For this review, take the finished solid that the model builds, in its own axes (mm). A direction names the side the tool comes from. Round coordinates to 2 decimals unless told otherwise and drop trailing zeros. Loops run counter-clockwise (first coordinate to the right, second up) from the corner with the lowest first, then second, coordinate; pieces in that order, holes last. Notation, with made-up numbers: (56, 58.25) -> (88, 58.25) arc R24 ccw to (88, 76.25) -> close; hole circle Ø5 at (68.25, 82). An arc over 180 degrees is marked (long way). Use one line per item in the form item = value. Start each with the question number.
from build123d import *

# Parameters (mm, degrees)
F1_DEPTH = 127
F2_W     = 101.6
F2_H     = 63.5
F3_DEPTH = 50.8


with BuildPart() as f1:
    # F0 (on Front) → F1 (new body)
    with BuildSketch(Plane.XZ):
        Polygon((-25.4, 95.645057), (-25.4, -5.954943), (127, -5.954943), (127, 95.645057), (101.6, 95.645057), (101.6, 44.845057), (0, 44.845057), (0, 95.645057), align=None)
    extrude(amount=F1_DEPTH)

    # F2 (on face) → F3 (join)
    with BuildSketch(Plane.XY.offset(44.845057)):
        with Locations((50.8, -31.75)):
            Rectangle(F2_W, F2_H)
    extrude(amount=F3_DEPTH)


solid = f1.part
Item 1: For P1, Ø5, axis at x = 72.5, z = 20.5, coming from the +Y side, flat-tipped, find the tip position at first contact; note if it passes through.
Item 2: Draft analysis for pull direction X (two halves, no side actions). For faces 1 (the flat face through (52, -95, 44.845)), 2 (the flat face through (50, -48, 95.645)), 3 (the flat face through (-25.4, -63, 46)), 4 (the flat face through (50, -63.5, 70)), state which applies: +X half, -X half, draft (parallel to the pull), parting line (faces both ways), or undercut.
Item 3: Wall thickness on line 1 (X direction, y = -95, z = 73); line 2 (Y direction, x = 92.5, z = 58); line 3 (Z direction, x = 63, y = -109): over which ranges is each line inside the solid? List them lowest first.
Item 4: Machinability: for faces 5 (the flat face through (0, -95, 70)), 6 (the flat face through (50, -63, -5.955)), which of the approach directions +Z, -Z, +X, -X, +Y, -Y give a long, thin tool a straight path to every point of the face, cutting with its end or side? Answer none if there is none.
Item 5: Take a section at A-A on y = -98.5. Give the boundary of the cut face in (x, z).
Item 6: Take a section at B-B on z = 69.5. Give the boundary of the cut face in (x, y), plus the area to 3 significant figures.
Item 7: Take a section at C-C on x = 35. Give the boundary of the cut face in (y, z).
Results:
q1.P1 = 0
q2.face_1 = undercut
q2.face_2 = draft
q2.face_3 = -X half
q2.face_4 = undercut
q3.line_1 = -25.4 to 0, 101.6 to 127
q3.line_2 = -63.5 to 0
q3.line_3 = -5.95 to 44.85
q4.face_5 = +Z, -Y
q4.face_6 = -Z, +X, -X, +Y, -Y
q5.outline = (-25.4, -5.95) -> (127, -5.95) -> (127, 95.65) -> (101.6, 95.65) -> (101.6, 44.85) -> (0, 44.85) -> (0, 95.65) -> (-25.4, 95.65) -> close
q6.outline = (-25.4, -127) -> (0, -127) -> (0, -63.5) -> (101.6, -63.5) -> (101.6, -127) -> (127, -127) -> (127, 0) -> (-25.4, 0) -> close
q6.area = 12,900 mm2
q7.outline = (-127, -5.95) -> (0, -5.95) -> (0, 95.65) -> (-63.5, 95.65) -> (-63.5, 44.85) -> (-127, 44.85) -> close
